```python
from build123d import *

# Parameters (mm, degrees)
SKETCH_1_W             = 130
SKETCH_1_H             = 90
EXTRUDE_1_DEPTH        = 10
SKETCH_2_W             = 22
SKETCH_2_H             = 28
CUT_EXTRUDE_1_DEPTH    = 8
SKETCH_3_W             = 25
SKETCH_3_H             = 6
CUT_EXTRUDE_2_DEPTH    = 131
EXTRUDE_2_DEPTH        = 130
SKETCH_7_R             = 2.5
CUT_EXTRUDE_5_DEPTH    = 9
SKETCH_5_R             = 1
CUT_EXTRUDE_6_DEPTH    = 131
CUT_EXTRUDE_8_DEPTH    = 18
PATTERN_LINEAR_1_COUNT = 4
PATTERN_LINEAR_1_PITCH = 24
CUT_EXTRUDE_9_DEPTH    = 0.5
PATTERN_LINEAR_2_COUNT = 4
PATTERN_LINEAR_2_PITCH = 24
MIRROR_1_COPY_1_DEPTH  = 0.5
MIRROR_1_COPY_2_DEPTH  = 0.5
MIRROR_1_COPY_3_DEPTH  = 0.5
SKETCH_11_W            = 86
SKETCH_11_H            = 8
CUT_EXTRUDE_10_DEPTH   = 32
SKETCH_12_W            = 30.395595504
SKETCH_12_H            = 8
CUT_EXTRUDE_11_DEPTH   = 8


with BuildPart() as part:
    # 草图1 → 凸台-拉伸1 (new body)
    with BuildSketch(Plane(origin=(0, 0, 0), x_dir=(1, 0, 0), z_dir=(0, 1, 0))):
        with Locations((65, 45)):
            Rectangle(SKETCH_1_W, SKETCH_1_H)
    extrude(amount=EXTRUDE_1_DEPTH)

    # 草图2 → 切除-拉伸1 (cut)
    with BuildSketch(Plane(origin=(0, 10, 0), x_dir=(1, 0, 0), z_dir=(0, 1, 0))):
        with Locations((13, 74)):
            Rectangle(SKETCH_2_W, SKETCH_2_H)
        with Locations((37, 74)):
            Rectangle(SKETCH_2_W, SKETCH_2_H)
        with Locations((61, 74)):
            Rectangle(SKETCH_2_W, SKETCH_2_H)
        with Locations((85, 74)):
            Rectangle(SKETCH_2_W, SKETCH_2_H)
        with Locations((37, 16)):
            Rectangle(SKETCH_2_W, SKETCH_2_H)
        with Locations((61, 16)):
            Rectangle(SKETCH_2_W, SKETCH_2_H)
        with Locations((85, 16)):
            Rectangle(SKETCH_2_W, SKETCH_2_H)
        with Locations((13, 16)):
            Rectangle(SKETCH_2_W, SKETCH_2_H)
    extrude(amount=-CUT_EXTRUDE_1_DEPTH, mode=Mode.SUBTRACT)

    # 草图3 → 切除-拉伸2 (cut, through all)
    with BuildSketch(Plane.ZY):
        with Locations((-45, 3)):
            Rectangle(SKETCH_3_W, SKETCH_3_H)
    extrude(amount=-CUT_EXTRUDE_2_DEPTH, mode=Mode.SUBTRACT)

    # 草图4 → 凸台-拉伸2 (add, through all)
    with BuildSketch(Plane.ZY):
        with BuildLine():
            Line((-49, 10), (-41, 10))
            ThreePointArc((-41, 10), (-45, 14), (-49, 10))
        make_face()
    extrude(amount=-EXTRUDE_2_DEPTH)

    # 草图7 → 切除-拉伸5 (cut, through all)
    with BuildSketch(Plane.XZ.offset(-6)):
        with Locations((13, -36.5)):
            Circle(SKETCH_7_R)
        with Locations((37, -36.5)):
            Circle(SKETCH_7_R)
        with Locations((61, -36.5)):
            Circle(SKETCH_7_R)
        with Locations((85, -36.5)):
            Circle(SKETCH_7_R)
        with Locations((85, -53.5)):
            Circle(SKETCH_7_R)
        with Locations((61, -53.5)):
            Circle(SKETCH_7_R)
        with Locations((37, -53.5)):
            Circle(SKETCH_7_R)
        with Locations((13, -53.5)):
            Circle(SKETCH_7_R)
    extrude(amount=-CUT_EXTRUDE_5_DEPTH, mode=Mode.SUBTRACT)

    # 草图5 → 切除-拉伸6 (cut, through all)
    with BuildSketch(Plane.ZY):
        with Locations((-45, 12)):
            Circle(SKETCH_5_R)
    extrude(amount=-CUT_EXTRUDE_6_DEPTH, mode=Mode.SUBTRACT)

    # 草图8 → 切除-拉伸8 (cut)
    with BuildSketch(Plane.ZY.offset(-4)):
        Polygon((-49, 10), (-49, 15.914476158), (-40.761753379, 15.914476158), (-41, 10), align=None)
    cut_extrude_8 = extrude(amount=-CUT_EXTRUDE_8_DEPTH, mode=Mode.SUBTRACT)

    # 阵列(线性)1: 切除-拉伸8 ×4
    with Locations(*[(i * PATTERN_LINEAR_1_PITCH, 0, 0) for i in range(1, PATTERN_LINEAR_1_COUNT)]):
        add(cut_extrude_8, mode=Mode.SUBTRACT)

    # 草图10 → 切除-拉伸9 (cut)
    with BuildSketch(Plane(origin=(0, 0, -90), x_dir=(-1, 0, 0), z_dir=(0, 0, -1))):
        Polygon((-12.992503856, 7.1), (-11.792503856, 7.1), (-11.792503856, 5.9), (-13.082457584, 5.9), (-14.282457584, 5.9), (-14.282457584, 7.1), align=None)
    cut_extrude_9 = extrude(amount=-CUT_EXTRUDE_9_DEPTH, mode=Mode.SUBTRACT)

    # 阵列(线性)2: 切除-拉伸9 ×4
    with Locations(*[(i * PATTERN_LINEAR_2_PITCH, 0, 0) for i in range(1, PATTERN_LINEAR_2_COUNT)]):
        add(cut_extrude_9, mode=Mode.SUBTRACT)

    # 镜向1: 切除-拉伸9 across plane
    add(cut_extrude_9.mirror(Plane.XY.offset(-44.896142346)), mode=Mode.SUBTRACT)

    # 镜向1 copy 1 sketch → 镜向1 copy 1 (cut)
    with BuildSketch(Plane(origin=(24, 0, 0.207715309), x_dir=(-1, 0, 0), z_dir=(0, 0, 1))):
        Polygon((-12.992503856, -7.1), (-11.792503856, -7.1), (-11.792503856, -5.9), (-13.082457584, -5.9), (-14.282457584, -5.9), (-14.282457584, -7.1), align=None)
    extrude(amount=-MIRROR_1_COPY_1_DEPTH, mode=Mode.SUBTRACT)

    # 镜向1 copy 2 sketch → 镜向1 copy 2 (cut)
    with BuildSketch(Plane(origin=(48, 0, 0.207715309), x_dir=(-1, 0, 0), z_dir=(0, 0, 1))):
        Polygon((-12.992503856, -7.1), (-11.792503856, -7.1), (-11.792503856, -5.9), (-13.082457584, -5.9), (-14.282457584, -5.9), (-14.282457584, -7.1), align=None)
    extrude(amount=-MIRROR_1_COPY_2_DEPTH, mode=Mode.SUBTRACT)

    # 镜向1 copy 3 sketch → 镜向1 copy 3 (cut)
    with BuildSketch(Plane(origin=(72, 0, 0.207715309), x_dir=(-1, 0, 0), z_dir=(0, 0, 1))):
        Polygon((-12.992503856, -7.1), (-11.792503856, -7.1), (-11.792503856, -5.9), (-13.082457584, -5.9), (-14.282457584, -5.9), (-14.282457584, -7.1), align=None)
    extrude(amount=-MIRROR_1_COPY_3_DEPTH, mode=Mode.SUBTRACT)

    # 草图11 → 切除-拉伸10 (cut)
    with BuildSketch(Plane(origin=(130, 0, 0), x_dir=(0, 0, -1), z_dir=(1, 0, 0))):
        with Locations((45, 4)):
            Rectangle(SKETCH_11_W, SKETCH_11_H)
    extrude(amount=-CUT_EXTRUDE_10_DEPTH, mode=Mode.SUBTRACT)

    # 草图12 → 切除-拉伸11 (cut)
    with BuildSketch(Plane(origin=(0, 10, 0), x_dir=(1, 0, 0), z_dir=(0, 1, 0))):
        with Locations((114.802202248, 45)):
            Rectangle(SKETCH_12_W, SKETCH_12_H)
    extrude(amount=CUT_EXTRUDE_11_DEPTH, mode=Mode.SUBTRACT)


solid = part.part
```
The model under review builds one solid part; all positions refer to its coordinate system, in mm. A direction names the side the tool comes from. Give positions to 0.01 mm unless a question says otherwise; leave off trailing zeros. Write each loop counter-clockwise with the first axis right and the second up, starting at its lowest first coordinate (ties: lowest second). Pieces come first, ordered by that corner, then holes. Notation, with made-up numbers: M 19,-7 L 62,-7 A27 cw 62,25 Z; hole C 69.25,-21 d9. An arc over 180 degrees is marked long. Write item = value, one per line. Start each with the question number.
Q1. We need section A-A (y = 3.5). Give the number of separate pieces and of enclosed holes in the cut face, plus the area to 3 significant figures.
Q2. We need section C-C (x = 79). State the section outline as (y, z) points.
Q3. Machinability: for faces 1 (the face through (64, 5, -90)), 2 (the face through (94, 10.7, -44.9)), 3 (the face through (114, 8, -44)), 4 (the face through (13, 6, -60)), which of the approach directions +Z, -Z, +X, -X, +Y, -Y give a long, thin tool a straight path to every point of the face, cutting with its end or side? Answer none if there is none.
Q4. Clearance check with flat-ended pins moving along their axes: pin 1 (3 mm diameter, centred on x = 38, y = 3.5, fed in from +Z); pin 2 (2 mm diameter, centred on x = 26, y = 12.5, fed in from -Z); pin 3 (2.5 mm diameter, centred on y = 6.5, z = -69, fed in from +X); pin 4 (1.5 mm diameter, centred on x = 48, z = -46.5, fed in from -Y). State where each tip first meets the part, or that it passes through.
Q5. For line 1 (X direction, y = 5.25, z = -62); line 2 (Z direction, x = 35, y = 3); line 3 (Z direction, x = 37, y = 8.5), list the stretches that pass through material, from the lowest coordinate up.
Q6. We need section B-B (z = -13). State the section outline as (x, y) points.
Q7. Mouldability with a two-part tool opening along X and no side actions: class faces 5 (the face through (82.5, 8, -53.4)), 6 (the face through (97, 14, -45)), 7 (the face through (39.31, 7.97, -54.46)) as released by +X, released by -X, zero draft, split by the parting line, or undercut.
Result set:
q1.separate_pieces = 2
q1.enclosed_holes = 8
q1.area = 1,570 mm2
q2.outline = M 0,-90 L 10,-90 L 10,-88 L 2,-88 L 2,-60 L 10,-60 L 10,-30 L 2,-30 L 2,-2 L 10,-2 L 10,0 L 0,0 L 0,-32.5 L 6,-32.5 L 6,-57.5 L 0,-57.5 Z
q3.face_1 = -Z, +X, -X, +Y, -Y
q3.face_2 = +Z, -Z, +Y
q3.face_3 = +X, -Y
q3.face_4 = +Y
q4.pin_1 = 0
q4.pin_2 = -48.71
q4.pin_3 = 98
q4.pin_4 = 6
q5.line_1 = 0 to 2, 24 to 26, 48 to 50, 72 to 74, 96 to 98
q5.line_2 = -90 to -88, -60 to -57.5, -32.5 to -30, -2 to 0
q5.line_3 = -90 to -88, -60 to -56, -51 to -39, -34 to -30, -2 to 0
q6.outline = M 0,0 L 98,0 L 98,8 L 130,8 L 130,10 L 96,10 L 96,2 L 74,2 L 74,10 L 72,10 L 72,2 L 50,2 L 50,10 L 48,10 L 48,2 L 26,2 L 26,10 L 24,10 L 24,2 L 2,2 L 2,10 L 0,10 Z
q7.face_5 = undercut
q7.face_6 = zero draft
q7.face_7 = undercut
